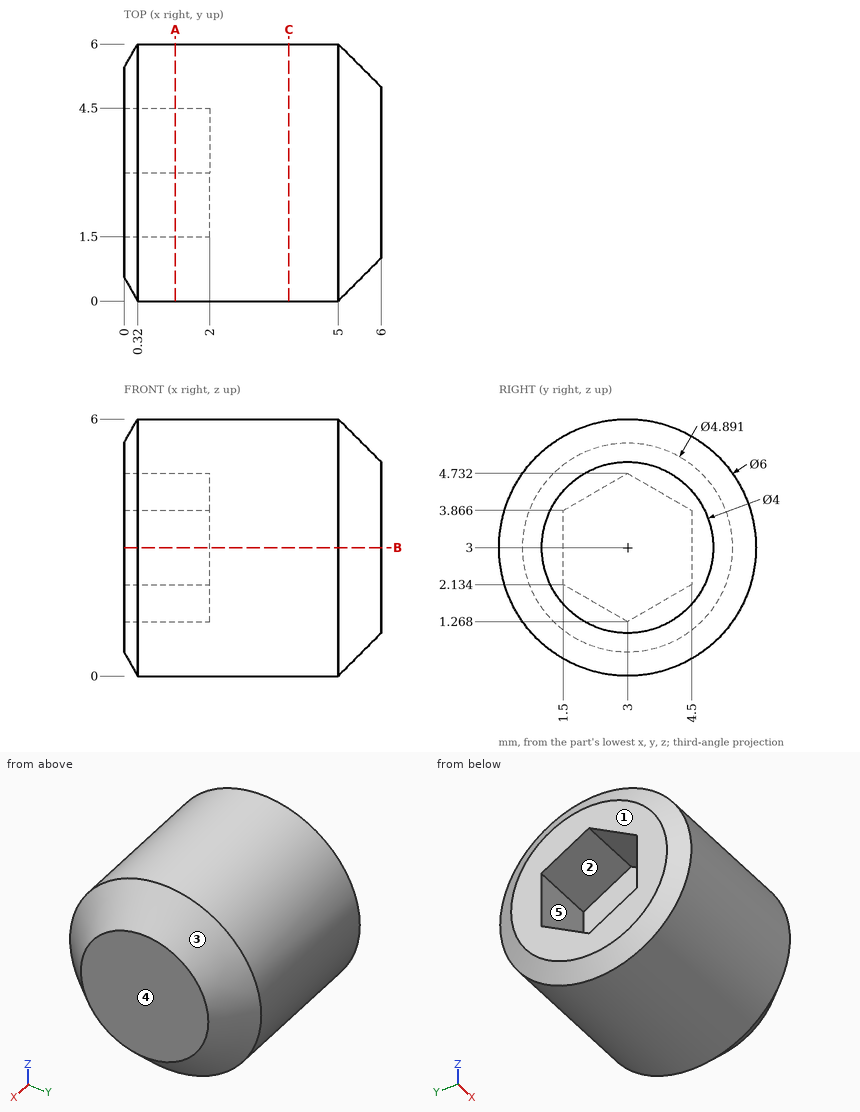
Could you check a few things on this drawing? It's one solid part, dimensions in mm from its lowest x, y, z. A direction names the side the tool comes from. Coordinates: 2 decimals unless noted, no trailing zeros. Loops run counter-clockwise (first coordinate to the right, second up) from the corner with the lowest first, then second, coordinate; pieces in that order, holes last. Notation, with made-up numbers: (75.5, 76) - (82.5, 76) arc R28 cw to (82.5, 95) - close; hole circle Ø10 at (-33, 59). An arc over 180 degrees is marked (long way). Answer as a JSON object with one key per item and string values. Group by question number.
Item 1: If we section it at C-C (x = 3.85): List the corners of the cut face in (y, z) for me, plus the area to 3 significant figures.
Item 2: If we section it at A-A (x = 1.2): List the corners of the cut face in (y, z) for me.
Item 3: For pin 1 (2 mm diameter, centred on x = 3.5, z = 1.5, fed in from +Y); pin 2 (0.5 mm diameter, centred on x = 1.5, z = 2.5, fed in from -Y), each with a flat end and sliding along its axis, tell me the tip position at first contact or that it passes through.
Item 4: If we section it at B-B (z = 3): List the corners of the cut face in (x, y) for me.
Item 5: On a 3-axis mill with a long thin cutter (end or side, diameter ignored), from which of +Z, -Z, +X, -X, +Y, -Y can I reach the whole of each face in a straight line? I mean the marked faces 1 and 2. Say none if no direction works.
Item 6: If I drill on L1, parallel to X at y = 2.35, z = 2.6; L2, parallel to Z at x = 0.45, y = 1.95; L3, parallel to Y at x = 1.2, z = 4.4 (1 decimal), over which ranges is the centre line in solid material (lowest first)? Write a range as from..to.
Item 7: If we mould it in two halves opening along Z, with no side actions, what happens to the marked faces 3, 4 and 5? For each: released by +Z, released by -Z, zero draft, split by the parting line, or undercut.
Returned:
{
 "1": {"outline": "circle Ø6 at (3, 3)", "area": "28.3 mm²"},
 "2": {"outline": "circle Ø6 at (3, 3); hole (1.5, 2.13) - (3, 1.27) - (4.5, 2.13) - (4.5, 3.87) - (3, 4.73) - (1.5, 3.87) - close"},
 "3": {"pin 1": "stops at y = 5.96", "pin 2": "stops at y = 0.01"},
 "4": {"outline": "(0, 0.55) - (0.32, 0) - (5, 0) - (6, 1) - (6, 5) - (5, 6) - (0.32, 6) - (0, 5.45) - (0, 4.5) - (2, 4.5) - (2, 1.5) - (0, 1.5) - close"},
 "5": {"face 1": "+Z, -Z, -X, +Y, -Y", "face 2": "-X"},
 "6": {"L1": "x = 2..6", "L2": "z = 0.19..1.87, 4.13..5.81", "L3": "y = 0.3..2.4, 3.6..5.7"},
 "7": {"face 3": "split by the parting line", "face 4": "zero draft", "face 5": "undercut"}
}
